```python
from build123d import *

# Parameters (mm, degrees)
SKETCH1_W            = 127.6
SKETCH1_H            = 85.5
BOSS_EXTRUDE1_DEPTH  = 14.4
SKETCH2_W            = 127.6
SKETCH2_H            = 85.5
SKETCH2_W_2          = 123.5
SKETCH2_H_2          = 81.2
CUT_EXTRUDE1_DEPTH   = 11.7
FILLET1_R            = 0.5
SKETCH3_R            = 3.4
CUT_EXTRUDE2_DEPTH   = 9.8
LPATTERN2_COUNT      = 8
LPATTERN2_PITCH      = 9
LPATTERN2_COUNT_DIR2 = 12
LPATTERN2_PITCH_DIR2 = 9
CUT_EXTRUDE3_DEPTH   = 11.7
FILLET2_R            = 0.5


with BuildPart() as part:
    # Sketch1 → Boss-Extrude1 (new body)
    with BuildSketch(Plane.XY):
        Rectangle(SKETCH1_W, SKETCH1_H)
    extrude(amount=BOSS_EXTRUDE1_DEPTH)

    # Sketch2 → Cut-Extrude1 (cut)
    with BuildSketch(Plane(origin=(0, 0, 0), x_dir=(-1, 0, 0), z_dir=(0, 0, -1))):
        Rectangle(SKETCH2_W, SKETCH2_H)
        Rectangle(SKETCH2_W_2, SKETCH2_H_2, mode=Mode.SUBTRACT)
    extrude(amount=-CUT_EXTRUDE1_DEPTH, mode=Mode.SUBTRACT)

    # Fillet1
    fillet1_edges = [part.edges().sort_by_distance(p)[0] for p in [
        (-61.75, -40.6, 5.85),
        (61.75, -40.6, 5.85),
        (61.75, 40.6, 5.85),
        (-61.75, 40.6, 5.85),
        (63.8, -42.75, 13.05),
        (-63.8, -42.75, 13.05),
        (-63.8, 42.75, 13.05),
        (63.8, 42.75, 13.05),
    ]]
    fillet(fillet1_edges, radius=FILLET1_R)

    # Sketch3 → Cut-Extrude2 (cut)
    with BuildSketch(Plane(origin=(0, 0, 0), x_dir=(-1, 0, 0), z_dir=(0, 0, -1))):
        with Locations((-49.4, 31.35)):
            Circle(SKETCH3_R)
    cut_extrude2 = extrude(amount=-CUT_EXTRUDE2_DEPTH, mode=Mode.SUBTRACT)

    # LPattern2: Cut-Extrude2 8 × 12
    with Locations(*[(-j * LPATTERN2_PITCH_DIR2, -i * LPATTERN2_PITCH, 0) for i in range(LPATTERN2_COUNT) for j in range(LPATTERN2_COUNT_DIR2) if (i, j) != (0, 0)]):
        add(cut_extrude2, mode=Mode.SUBTRACT)

    # Sketch4 → Cut-Extrude3 (cut)
    with BuildSketch(Plane(origin=(0, 0, 0), x_dir=(-1, 0, 0), z_dir=(0, 0, -1))):
        Polygon((-64.33792147, -30.250790597), (-51.805815692, -42.782896374), (-64.33792147, -42.782896374), align=None)
        Polygon((64.33792147, -42.782896374), (64.33792147, -30.250790597), (51.805815692, -42.782896374), align=None)
    extrude(amount=-CUT_EXTRUDE3_DEPTH, mode=Mode.SUBTRACT)

    # Fillet2
    fillet2_edges = [part.edges().sort_by_distance(p)[0] for p in [
        (53.988712066, -40.6, 5.85),
        (61.75, -32.838712066, 5.85),
        (-61.75, -32.838712066, 5.85),
        (-53.988712066, -40.6, 5.85),
    ]]
    fillet(fillet2_edges, radius=FILLET2_R)


solid = part.part
```
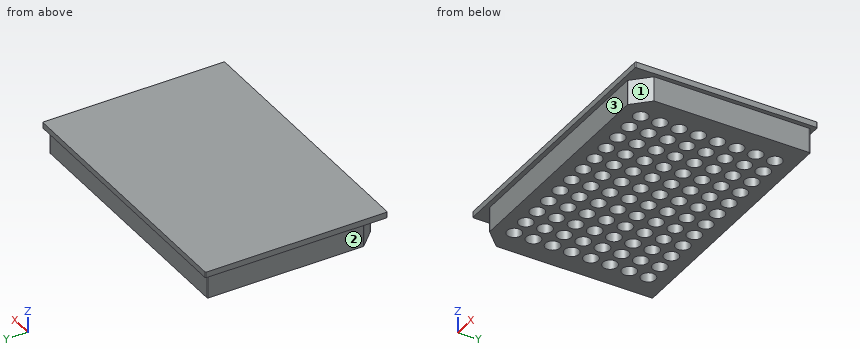
For this review, take the finished solid that the model builds, in its own axes (mm). Face numbers are marked on the shaded views. A direction names the side the tool comes from. Give positions to 0.01 mm unless a question says otherwise; leave off trailing zeros. One line per item, written item: value. Start each with the question number.
Q1. Add section A-A (z = 1.25). Count the separate pieces of the cut face and the enclosed holes in it, and give its area (3 significant figures).
Q2. For L1, parallel to Z at x = 40.5, y = 12; L2, parallel to Y at x = 29, z = 11.25; L3, parallel to X at y = 0.5, z = 10.75, list the stretches that pass through material, from the lowest coordinate up.
Q3. Machinability: for the marked faces 1, 2 and 3, which of the approach directions +Z, -Z, +X, -X, +Y, -Y give a long, thin tool a straight path to every point of the face, cutting with its end or side? Answer none if there is none.
Q4. Clearance check with flat-ended pins moving along their axes: pin 1 Ø2 at (x, z) = (26.5, 7.5) entering from -Y; pin 2 Ø3.5 at (x, y) = (-22.5, -5.5) entering from -Z; pin 3 Ø1.5 at (x, z) = (-49.5, 5.5) entering from +Y. State where each tip first meets the part, or that it passes through.
Reply:
1. separate pieces: 1
1. enclosed holes: 96
1. area: 6,480 mm²
2. L1: 9.8 to 14.4
2. L2: -40.6 to 40.6
2. L3: -61.75 to 61.75
3. face 1: -Z, +X, -Y
3. face 2: -Z, -X, +Y, -Y
3. face 3: -Z, +X, -X, -Y
4. pin 1: y = -40.6
4. pin 2: z = 9.8
4. pin 3: y = 40.6
